Source: CAD feature listing. Evaluate the final solid. Frame: model axes, mm. Face numbers are marked on the shaded views. A direction names the side the tool comes from. Give positions to 0.01 mm unless a question says otherwise; leave off trailing zeros. Loops run counter-clockwise (first coordinate to the right, second up) from the corner with the lowest first, then second, coordinate; pieces in that order, holes last. Notation, with made-up numbers: (89, -23) -> (117, -23) arc R21 cw to (117, 7) -> close; hole circle Ø8 at (20.25, -0.75). An arc over 180 degrees is marked (long way). Put each result on its own line as item: value.
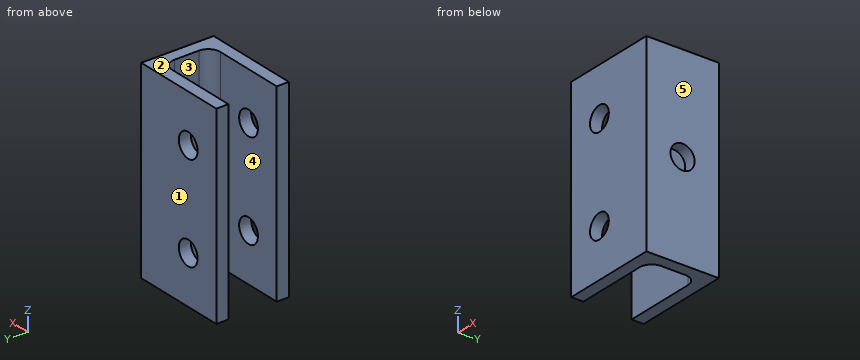
```python
from build123d import *

# Parameters (mm, degrees)
BOSS_EXTRUDE1_DEPTH = 80
FILLET1_R           = 5
SKETCH2_R           = 5
CUT_EXTRUDE1_DEPTH  = 75
SKETCH3_R           = 5
CUT_EXTRUDE2_DEPTH  = 10


with BuildPart() as part:
    # Sketch1 → Boss-Extrude1 (new body)
    with BuildSketch(Plane.XY):
        Polygon((0, 0), (35, 0), (35, -20), (0, -20), (0, -25), (40, -25), (40, 5), (0, 5), align=None)
    extrude(amount=BOSS_EXTRUDE1_DEPTH)

    # Fillet1
    fillet1_edges = [part.edges().sort_by_distance(p)[0] for p in [
        (35, -20, 40),
        (35, 0, 40),
    ]]
    fillet(fillet1_edges, radius=FILLET1_R)

    # Sketch2 → Cut-Extrude1 (cut)
    with BuildSketch(Plane(origin=(0, 5, 0), x_dir=(1, 0, 0), z_dir=(0, 1, 0))):
        with Locations(Location((15, -60, 0), (0, 0, 180))):
            Circle(SKETCH2_R)
        with Locations(Location((15, -20, 0), (0, 0, 270))):
            Circle(SKETCH2_R)
    extrude(amount=-CUT_EXTRUDE1_DEPTH, mode=Mode.SUBTRACT)

    # Sketch3 → Cut-Extrude2 (cut)
    with BuildSketch(Plane(origin=(40, 0, 0), x_dir=(0, 0, -1), z_dir=(1, 0, 0))):
        with Locations((-40, -10)):
            Circle(SKETCH3_R)
    extrude(amount=-CUT_EXTRUDE2_DEPTH, mode=Mode.SUBTRACT)


solid = part.part
```
(1) Draft query along Y for the marked faces 1, 2 and 3. Return one class per face: released by +Y, released by -Y, zero draft, split by the parting line, or undercut.
Calculated:
face 1: released by +Y
face 2: zero draft
face 3: undercut
(2) Section C-C on y = 2.5. Return loops of the section in (x, z).
Calculated:
outline: (0, 0) -> (40, 0) -> (40, 80) -> (0, 80) -> close; hole circle Ø10 at (15, 20); hole circle Ø10 at (15, 60)
(3) Reachability of the marked faces 4 and 5 from +Z, -Z, +X, -X, +Y, -Y: full face, straight path, thin tool, end or side. Return the list, or none.
Calculated:
face 4: +Z, -Z, -X
face 5: +Z, -Z, +X, +Y, -Y
(4) Section A-A on z = 60. Return loops of the section in (x, y).
Calculated:
outline: (0, -25) -> (10, -25) -> (10, -20) -> (0, -20) -> close; (0, 0) -> (10, 0) -> (10, 5) -> (0, 5) -> close; (20, -25) -> (40, -25) -> (40, 5) -> (20, 5) -> (20, 0) -> (30, 0) arc R5 cw to (35, -5) -> (35, -15) arc R5 cw to (30, -20) -> (20, -20) -> close
(5) Line query: probe 1 along Y at (x, z) = (15.5, 69); probe 2 along Y at (x, z) = (38.6, 40); probe 3 along Z at (x, y) = (38.75, -10). Output: solid intervals per line, ascending. Write a range as from..to.
Calculated:
probe 1: y = -25..-20, 0..5
probe 2: y = -25..-15, -5..5
probe 3: z = 0..35, 45..80
(6) First-contact query: P1, Ø8, axis at y = -10.5, z = 68.5, coming from the -X side; P2, Ø11, axis at y = -7.5, z = 28, coming from the -X side. Flat tips, straight axial feed; report the tip coordinate or a pass-through.
Calculated:
P1: stops at x = 35
P2: stops at x = 34
(7) Section D-D on z = 43.5. Return loops of the section in (x, y).
Calculated:
outline: (0, -25) -> (40, -25) -> (40, -13.57) -> (35, -13.57) -> (35, -15) arc R5 cw to (30, -20) -> (0, -20) -> close; (0, 0) -> (30, 0) arc R5 cw to (35, -5) -> (35, -6.43) -> (40, -6.43) -> (40, 5) -> (0, 5) -> close
(8) Section B-B on x = 26.5. Return loops of the section in (y, z), then the cut area to 3 significant figures.
Calculated:
outline: (-25, 0) -> (-20, 0) -> (-20, 80) -> (-25, 80) -> close; (0, 0) -> (5, 0) -> (5, 80) -> (0, 80) -> close
area: 800 mm²
